Can you work these out from the model? Positions are in its coordinate system, mm. Give positions to 0.01 mm unless a question says otherwise; leave off trailing zeros. Order: outer loops, then holes, each group sorted by start corner. A loop starts at its lowest first (then second) coordinate and runs counter-clockwise, first axis right, second up. Notation, with made-up numbers: M -22.5,-32 L 10.5,-32 A29 ccw 10.5,-11 Z; hole C 36,84.25 d6. An arc over 180 degrees is marked long. Use one line per item in the form item = value. Start each with the question number.
1. I need wall thicknesses on L1, parallel to X at y = 1, z = -328.5; L2, parallel to X at y = 0.5, z = -170.5; L3, parallel to X at y = -9, z = -346. Which ranges of each line are inside material? Lowest first, please.
2. I want a section at A-A, the plane z = -283.5. List the corners of the cut face in (x, y) for me, and give its area (3 significant figures).
3. Will these pins go through, and if not, where does the flat tip stop? P1, Ø1.5, axis at x = -3.5, y = -11, coming from the -Z side; P2, Ø5, axis at y = 4.5, z = -448, coming from the +X side; P3, Ø1.5, axis at x = -5.5, z = -473, coming from the -Y side; P4, Ø2, axis at y = -6.5, z = -383, coming from the +X side.
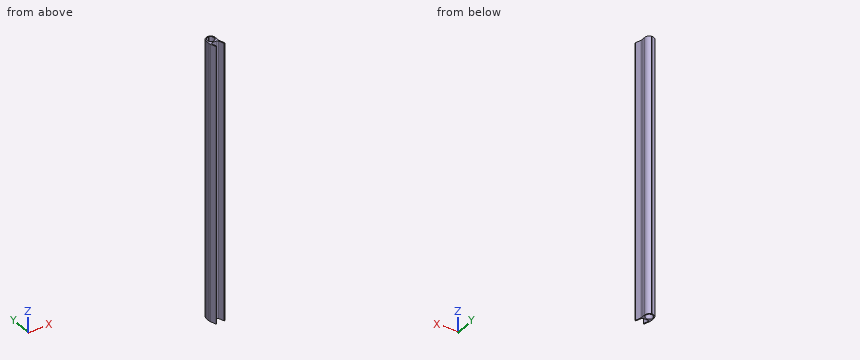
```python
from build123d import *

# Parameters (mm, degrees)
BOSS_EXTRUDE1_DEPTH = 580


with BuildPart() as part:
    # Sketch3 → Boss-Extrude1 (new body)
    with BuildSketch(Plane.XY):
        with BuildLine():
            Line((-6.034633842, -14.02606043), (-3.148633912, -21.955280071))
            ThreePointArc((-3.148633912, -21.955280071), (-3.746306389, -23.236992835), (-5.028019153, -22.639320358))
            Line((-5.028019153, -22.639320358), (-8.776311449, -12.340971913))
            ThreePointArc((-8.776311449, -12.340971913), (-9.317693036, -10.320508325), (-9.5, -8.236730193))
            Line((-9.5, -8.236730193), (-9.5, 0))
            ThreePointArc((-9.5, 0), (-6.488568374, 6.93891061), (0.636522201, 9.478651776))
            Line((0.636522201, 9.478651776), (0.502517527, 7.483146139))
            ThreePointArc((0.502517527, 7.483146139), (-5.12255398, 5.478087324), (-7.5, 0))
            ThreePointArc((-7.5, 0), (0, -7.5), (7.5, 0))
            ThreePointArc((7.5, 0), (5.645794895, 4.937104415), (1, 7.433034374))
            Line((1, 7.433034374), (1.266666667, 9.415176873))
            ThreePointArc((1.266666667, 9.415176873), (7.151340201, 6.253665592), (9.5, 0))
            Line((9.5, 0), (9.425154073, -8.236390129))
            ThreePointArc((9.425154073, -8.236390129), (9.540131353, -9.662460438), (9.907282817, -11.045246071))
            Line((9.907282817, -11.045246071), (13.878210448, -21.955280071))
            ThreePointArc((13.878210448, -21.955280071), (13.28053797, -23.236992835), (11.998825206, -22.639320358))
            Line((11.998825206, -22.639320358), (8.116944062, -11.97393957))
            ThreePointArc((8.116944062, -11.97393957), (7.018595509, -10.542543867), (5.2978662, -10))
            Line((5.2978662, -10), (-3.21555598, -10))
            ThreePointArc((-3.21555598, -10), (-5.673012113, -11.279270691), (-6.034633842, -14.02606043))
        make_face()
    extrude(amount=-BOSS_EXTRUDE1_DEPTH)


solid = part.part
```
Check result:
q1.L1 = -9.45 to -7.43, 7.43 to 9.45
q1.L2 = -9.49 to -7.48, 7.48 to 9.49
q1.L3 = -9.48 to 9.45
q2.outline = M -9.5,-8.24 A12 ccw -8.78,-12.34 L -5.03,-22.64 A1 ccw -3.15,-21.96 L -6.03,-14.03 A3 cw -3.22,-10 L 5.3,-10 A3 cw 8.12,-11.97 L 12,-22.64 A1 ccw 13.88,-21.96 L 9.91,-11.05 A8 cw 9.43,-8.24 L 9.5,0 A9.5 ccw 1.27,9.42 L 1,7.43 A7.5 cw long 0.5,7.48 L 0.64,9.48 A9.5 ccw -9.5,0 Z
q2.area = 214 mm2
q3.P1 = through
q3.P2 = 9.29
q3.P3 = -23.05
q3.P4 = 9.45
